Autodesk Inventor part; units mm, degrees
ref_plane "YZ Plane" through (0, 0, 0) normal (1, 0, 0) x (0, 1, 0)
ref_plane "XZ Plane" through (0, 0, 0) normal (0, 1, 0) x (-1, 0, 0)
ref_plane "XY Plane" through (0, 0, 0) normal (0, 0, 1) x (1, 0, 0)
sketch "Sketch1" plane through (0, 0, 0) normal (0, 1, 0) x (-1, 0, 0)
  line L0 (0, 0) -> (0, -100)
  arc A0 (93.6713, -124.5596) -> (117.8498, -82.8611) centre (100.0117, -100.377) ccw
  line L1 (0, -100) -> (93.6713, -124.5596)
  arc A1 (98.5447, -12.3594) -> (0, 0) centre (49.9985, -0.39) ccw
  arc A2 (99.0048, -10.5865) -> (117.8498, -82.8611) centre (171.3639, -30.3137) ccw
  arc A3 (49.1416, -75.3835) -> (49.6184, -45.3884) centre (49.5087, -60.388) ccw
  arc A4 (22.9948, -36.4248) -> (49.6184, -45.3884) centre (49.9477, -0.3896) ccw
  line L2 (15, -40.4287) -> (15, -70.4287)
  arc A5 (22.9948, -36.4248) -> (15, -40.4287) centre (20, -40.4287) ccw
  arc A6 (15, -70.4287) -> (29.3397, -79.438) centre (25, -70.4287) ccw
  arc A7 (49.1416, -75.3835) -> (29.1892, -79.5089) centre (48.0406, -120.37) ccw
  circle A8 centre (14.9985, 0) radius 5
  circle A9 centre (67.085, -30.8513) radius 5
  circle A10 centre (67.7598, 29.6826) radius 5
  dimension "d0" = 100
  dimension "d3" = 50
  dimension "d5" = 50
  dimension "d6" = 75
  dimension "d13" = 15
  dimension "d14" = 60
  dimension "d16" = 45
  dimension "d17" = 5
  dimension "d19" = 10
  dimension "d24" = 30
  dimension "d25" = 15
  dimension "d26" = 45
  dimension "d57" = 10
  dimension "d58" = 35
  dimension "d61" = 360
extrude "Extrusion2" add sketch "Sketch1" along normal blind 20
chamfer "Chamfer2" distance 2 angle 45 12 edges at (-64.5068, 20, -60.6264) (-38.9289, 20, -76.3021) (-19.6098, 20, -78.8516) (-15, 20, -55.4287) (-17.761, 20, -35.958) (-35.5892, 20, -43.0373) (-64.5068, 0, -60.6264) (-38.9289, 0, -76.3021) (-19.6098, 0, -78.8516) (-15, 0, -55.4287) (-17.761, 0, -35.958) (-35.5892, 0, -43.0373)
chamfer "Chamfer3" distance 0.5 angle 45 3 edges at (-62.085, 20, -30.8513) (-62.7598, 20, 29.6826) (-9.9985, 20, 0)
thread "Thread1"
thread "Thread2"
thread "Thread3"
properties part number "Curve"
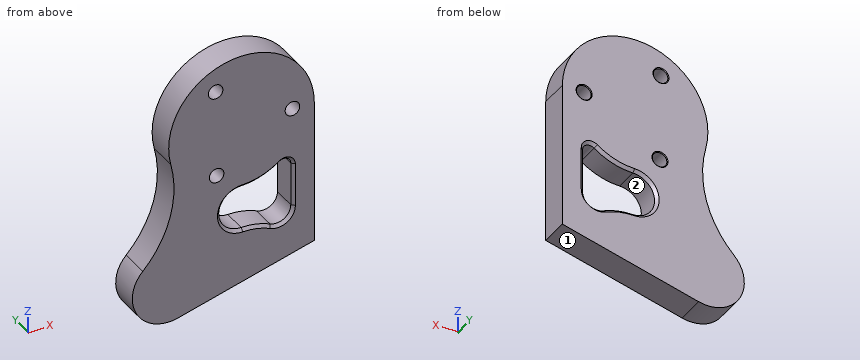
Work out the finished part from the listing and answer in its coordinate system (mm). Face numbers are marked on the shaded views. A direction names the side the tool comes from. Coordinates: 2 decimals unless noted, no trailing zeros. Loops run counter-clockwise (first coordinate to the right, second up) from the corner with the lowest first, then second, coordinate; pieces in that order, holes last.
1) Section C-C (z = 20.5) is taken. Give the vertices of the cut face in (x, y), plus the area to 3 significant figures.
Results:
outline: (-95.43, 0) - (-4.57, 0) - (-4.57, 20) - (-95.43, 20) - close
area: 1,820 mm2
2) Flat-ended cylindrical pins translate along their axes: pin 1 (1.5 mm diameter, centred on x = -33, y = 16.5, fed in from -Z); pin 2 (1 mm diameter, centred on x = -44, z = -28.5, fed in from -Y); pin 3 (10 mm diameter, centred on y = 17, z = -63.5, fed in from -X); pin 4 (5 mm diameter, centred on y = 10.5, z = -53, fed in from -X). Find the tip coordinate at first contact, or state that the pin passes through.
Results:
pin 1: stops at z = -108.85
pin 2: stops at y = 0
pin 3: stops at x = -106.81
pin 4: stops at x = -100.72
3) For the marked faces 1 and 2, determine the directions among +Z, -Z, +X, -X, +Y, -Y from which every point of the face is accessible in a straight line to the end or side of a thin tool.
Results:
face 1: -Z, +X, +Y, -Y
face 2: +Y, -Y
4) Consider probe 1 along Z at (x, y) = (-19, 5); probe 2 along Z at (x, y) = (-44, 2.25); probe 3 along Z at (x, y) = (-65, 15.5). Determine where each line is inside the solid, lowest interval first.
Results:
probe 1: z = -104.98 to -78.43, -35.53 to -3, 3 to 38.84
probe 2: z = -111.54 to -75.55, -44.99 to 49.25
probe 3: z = -117.04 to -35.4, -26.31 to 25.51, 33.85 to 47.31
5) Section A-A (y = 10) is taken. Give the vertices of the cut face in (x, z) (1 decimal), plus the area to 3 significant figures.
Results:
outline: (-117.8, -82.9) arc R25 ccw to (-93.7, -124.6) - (0, -100) - (0, 0) arc R50 ccw (long way) to (-98.5, -12.4) arc R75 cw to start; hole circle Ø10 at (-67.8, 29.7); hole circle Ø10 at (-67.1, -30.9); hole (-49.6, -45.4) arc R15 ccw (long way) to (-49.1, -75.4) arc R45 cw to (-29.3, -79.4) arc R10 ccw to (-15, -70.4) - (-15, -40.4) arc R5 ccw to (-23, -36.4) arc R45 cw to start; hole circle Ø10 at (-15, 0)
area: 14,300 mm2
6) Section B-B (x = -84.5) is taken. Give the vertices of the cut face in (y, z), plus the area to 3 significant figures.
Results:
outline: (0, -122.15) - (20, -122.15) - (20, 35.8) - (0, 35.8) - close
area: 3,160 mm2
